Study the drawing (mm; zero at the part's minimum x, y, z) and answer. Coordinates: 2 decimals unless noted, no trailing zeros. Write each loop counter-clockwise with the first axis right and the second up, starting at its lowest first coordinate (ties: lowest second). Pieces come first, ordered by that corner, then holes. Notation, with made-up numbers: (69, 71.5) - (75, 71.5) arc R22 ccw to (75, 104.5) - close; hole circle Ø10 at (18, -26). An arc over 180 degrees is marked (long way). One line per item, written item: value.
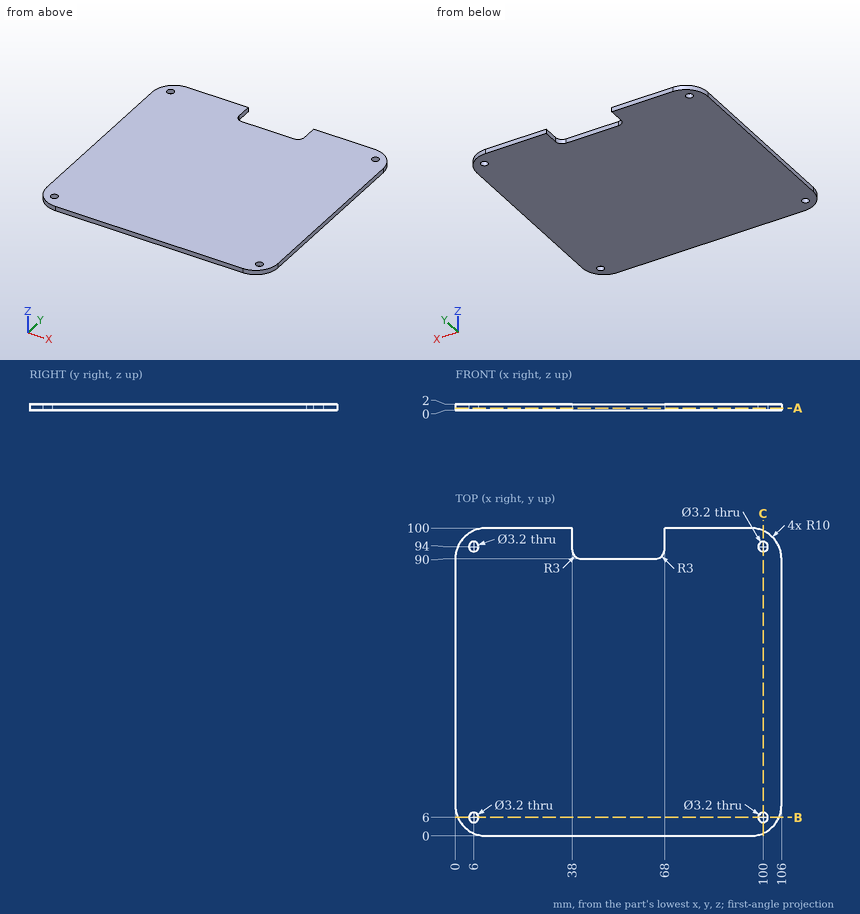
Item 1: Given pin 1 (2.5 mm diameter, centred on x = 6, y = 6, fed in from +Z); pin 2 (0.6 mm diameter, centred on x = 52, z = 0.5, fed in from +Y); pin 3 (1 mm diameter, centred on y = 97.5, z = 1, fed in from +X), each flat-ended and moving along its own axis, determine where each tip first touches the part or whether it passes through.
Evaluation:
pin 1: passes through
pin 2: stops at y = 90
pin 3: stops at x = 103.14
Item 2: Section A-A, the plane z = 0.7 is taken. Determine the outline of the cut face in (x, y).
Evaluation:
outline: (0, 10) arc R10 ccw to (10, 0) - (96, 0) arc R10 ccw to (106, 10) - (106, 90) arc R10 ccw to (96, 100) - (68, 100) - (68, 93) arc R3 cw to (65, 90) - (41, 90) arc R3 cw to (38, 93) - (38, 100) - (10, 100) arc R10 ccw to (0, 90) - close; hole circle Ø3.2 at (6, 6); hole circle Ø3.2 at (6, 94); hole circle Ø3.2 at (100, 6); hole circle Ø3.2 at (100, 94)
Item 3: Consider probe 1 along Y at (x, z) = (99.5, 0.95); probe 2 along Y at (x, z) = (6, 0.8); probe 3 along Y at (x, z) = (63, 1.85). Determine where each line is inside the solid, lowest interval first.
Evaluation:
probe 1: y = 0.63 to 4.48, 7.52 to 92.48, 95.52 to 99.37
probe 2: y = 0.83 to 4.4, 7.6 to 92.4, 95.6 to 99.17
probe 3: y = 0 to 90
Item 4: Section B-B, the plane y = 6 is taken. Determine the outline of the cut face in (x, z), then the cut area to 3 significant figures.
Evaluation:
outline: (0.83, 0) - (4.4, 0) - (4.4, 2) - (0.83, 2) - close; (7.6, 0) - (98.4, 0) - (98.4, 2) - (7.6, 2) - close; (101.6, 0) - (105.17, 0) - (105.17, 2) - (101.6, 2) - close
area: 196 mm2
Item 5: Section C-C, the plane x = 100 is taken. Determine the outline of the cut face in (y, z), then the cut area to 3 significant figures.
Evaluation:
outline: (0.83, 0) - (4.4, 0) - (4.4, 2) - (0.83, 2) - close; (7.6, 0) - (92.4, 0) - (92.4, 2) - (7.6, 2) - close; (95.6, 0) - (99.17, 0) - (99.17, 2) - (95.6, 2) - close
area: 184 mm2
